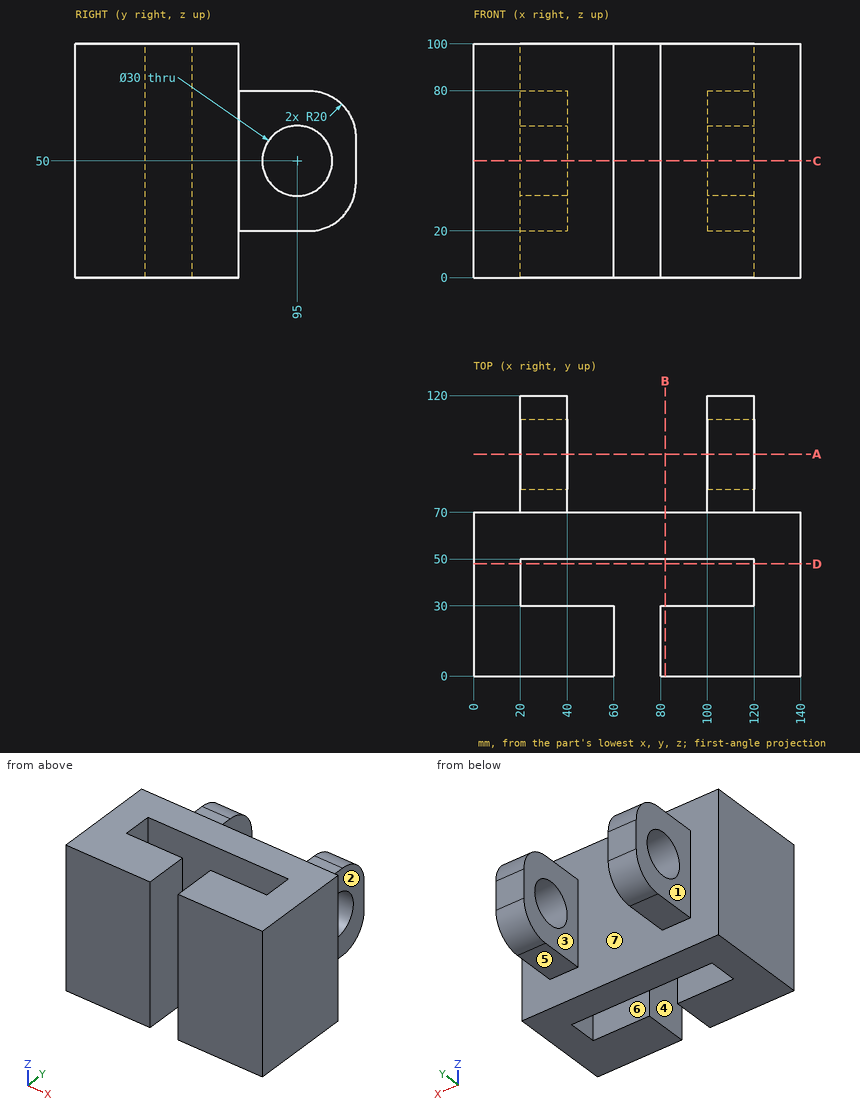
Design review of the part shown in the three views and the two pictorial views. Dimensions are in mm from the part's minimum x, y and z. A direction names the side the tool comes from. Round coordinates to 2 decimals unless told otherwise and drop trailing zeros. Write each loop counter-clockwise with the first axis right and the second up, starting at its lowest first coordinate (ties: lowest second). Pieces come first, ordered by that corner, then holes.
Item 1: For the marked faces 4, 5, 6 and 7, list the 3-axis set-ups (+Z, -Z, +X, -X, +Y, -Y) from which the entire face can be reached by the end or side of a thin tool; tool diameter is ignored.
Item 2: For probe 1 along Y at (x, z) = (110.25, 50); probe 2 along X at (y, z) = (43, 37); probe 3 along X at (y, z) = (11.5, 65.5), list the stretches that pass through material, from the lowest coordinate up.
Item 3: Clearance check with flat-ended pins moving along their axes: pin 1 Ø15 at (y, z) = (102, 62) entering from +X; pin 2 Ø16 at (x, y) = (106, 89.5) entering from +Z; pin 3 Ø25 at (y, z) = (94, 53) entering from -X. State where each tip first meets the part, or that it passes through.
Item 4: We need section D-D on y = 48. Write out the cut boundary in (x, z).
Item 5: We need section B-B on x = 82. Write out the cut boundary in (y, z).
Item 6: We need section C-C on z = 50. Write out the cut boundary in (x, y), and give its area (3 significant figures).
Item 7: The part is to be moulded in two halves that separate along X. For the marked faces 1, 2 and 3, say which applies: +X half, -X half, draft (parallel to the pull), parting line (faces both ways), or undercut.
Item 8: We need section A-A on y = 95. Write out the cut boundary in (x, z).
Returned:
1. face 4: +Z, -Z, -Y
1. face 5: -Z, +X, -X, +Y
1. face 6: +Z, -Z
1. face 7: +Y
2. probe 1: y = 0 to 30, 50 to 80, 110 to 120
2. probe 2: x = 0 to 20, 120 to 140
2. probe 3: x = 0 to 60, 80 to 140
3. pin 1: stops at x = 120
3. pin 2: stops at z = 80
3. pin 3: stops at x = 20
4. outline: (0, 0) - (20, 0) - (20, 100) - (0, 100) - close; (120, 0) - (140, 0) - (140, 100) - (120, 100) - close
5. outline: (0, 0) - (30, 0) - (30, 100) - (0, 100) - close; (50, 0) - (70, 0) - (70, 100) - (50, 100) - close
6. outline: (0, 0) - (60, 0) - (60, 30) - (20, 30) - (20, 50) - (120, 50) - (120, 30) - (80, 30) - (80, 0) - (140, 0) - (140, 70) - (120, 70) - (120, 80) - (100, 80) - (100, 70) - (40, 70) - (40, 80) - (20, 80) - (20, 70) - (0, 70) - close; (20, 110) - (40, 110) - (40, 120) - (20, 120) - close; (100, 110) - (120, 110) - (120, 120) - (100, 120) - close
6. area: 8,000 mm2
7. face 1: -X half
7. face 2: +X half
7. face 3: undercut
8. outline: (20, 20) - (40, 20) - (40, 35) - (20, 35) - close; (20, 65) - (40, 65) - (40, 80) - (20, 80) - close; (100, 20) - (120, 20) - (120, 35) - (100, 35) - close; (100, 65) - (120, 65) - (120, 80) - (100, 80) - close
